Verification items for the finished model (mm, model axes). Face numbers are marked on the shaded views. A direction names the side the tool comes from. Round coordinates to 2 decimals unless told otherwise and drop trailing zeros. Loops run counter-clockwise (first coordinate to the right, second up) from the corner with the lowest first, then second, coordinate; pieces in that order, holes last.
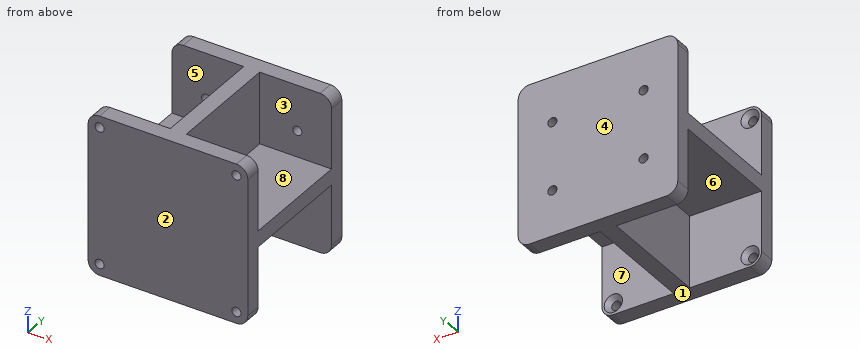
from build123d import *

# Parameters (mm, degrees)
SKETCH1_R           = 2
BOSS_EXTRUDE1_DEPTH = 3.5
BOSS_EXTRUDE2_DEPTH = 50
BOSS_EXTRUDE3_START = 7
SKETCH3_R           = 2
BOSS_EXTRUDE3_DEPTH = 7
CHAMFER1_SIZE       = 2


with BuildPart() as part:
    # Sketch1 → Boss-Extrude1 (new, symmetric)
    with BuildSketch(Plane(origin=(0, 0, 0), x_dir=(1, 0, 0), z_dir=(0, 1, 0))):
        with BuildLine():
            Line((-30, 35), (30, 35))
            ThreePointArc((30, 35), (33.535533906, 33.535533906), (35, 30))
            Line((35, 30), (35, -30))
            ThreePointArc((35, -30), (33.535533906, -33.535533906), (30, -35))
            Line((30, -35), (-30, -35))
            ThreePointArc((-30, -35), (-33.535533906, -33.535533906), (-35, -30))
            Line((-35, -30), (-35, 30))
            ThreePointArc((-35, 30), (-33.535533906, 33.535533906), (-30, 35))
        make_face()
        with Locations(Location((30, 30, 0), (0, 0, 270))):
            Circle(SKETCH1_R, mode=Mode.SUBTRACT)
        with Locations(Location((-30, 30, 0), (0, 0, 90))):
            Circle(SKETCH1_R, mode=Mode.SUBTRACT)
        with Locations(Location((30, -30, 0), (0, 0, 90))):
            Circle(SKETCH1_R, mode=Mode.SUBTRACT)
        with Locations(Location((-30, -30, 0), (0, 0, 270))):
            Circle(SKETCH1_R, mode=Mode.SUBTRACT)
    extrude(amount=BOSS_EXTRUDE1_DEPTH, both=True)

    # Sketch2 → Boss-Extrude2 (add)
    with BuildSketch(Plane(origin=(0, 3.5, 0), x_dir=(1, 0, 0), z_dir=(0, 1, 0))):
        Polygon((-3.5, 35), (3.5, 35), (3.5, 3.5), (35, 3.5), (35, -3.5), (3.5, -3.5), (3.5, -35), (-3.5, -35), (-3.5, -3.5), (-35, -3.5), (-35, 3.5), (-3.5, 3.5), align=None)
    extrude(amount=BOSS_EXTRUDE2_DEPTH)

    # Sketch3 → Boss-Extrude3 (add)
    with BuildSketch(Plane(origin=(0, 53.5, 0), x_dir=(1, 0, 0), z_dir=(0, 1, 0)).offset(BOSS_EXTRUDE3_START)):
        with BuildLine():
            Line((30, -35), (-30, -35))
            ThreePointArc((-30, -35), (-33.535533906, -33.535533906), (-35, -30))
            Line((-35, -30), (-35, 30))
            ThreePointArc((-35, 30), (-33.535533906, 33.535533906), (-30, 35))
            Line((-30, 35), (30, 35))
            ThreePointArc((30, 35), (33.535533906, 33.535533906), (35, 30))
            Line((35, 30), (35, -30))
            ThreePointArc((35, -30), (33.535533906, -33.535533906), (30, -35))
        make_face()
        with Locations(Location((20, -15, 0), (0, 0, 270))):
            Circle(SKETCH3_R, mode=Mode.SUBTRACT)
        with Locations(Location((20, 15, 0), (0, 0, 270))):
            Circle(SKETCH3_R, mode=Mode.SUBTRACT)
        with Locations(Location((-20, 15, 0), (0, 0, 90))):
            Circle(SKETCH3_R, mode=Mode.SUBTRACT)
        with Locations(Location((-20, -15, 0), (0, 0, 90))):
            Circle(SKETCH3_R, mode=Mode.SUBTRACT)
    extrude(amount=-BOSS_EXTRUDE3_DEPTH)

    # Chamfer1
    chamfer1_edges = [part.edges().sort_by_distance(p)[0] for p in [
        (30, 3.5, -32),
        (-30, 3.5, -28),
        (30, 3.5, 32),
        (-30, 3.5, 28),
    ]]
    chamfer(chamfer1_edges, length=CHAMFER1_SIZE)


solid = part.part
1. Release check for a two-part mould opening along Y. For the marked faces 1, 2, 3 and 4 record: released by +Y, released by -Y, zero draft, split by the parting line, or undercut.
2. Section check B-B (z = 15). Enter the section's corners in (x, y), then the cut area to 3 significant figures.
3. Scan lines: L1, parallel to Z at x = -20, y = 57.25; L2, parallel to X at y = -0.95, z = 30; L3, parallel to X at y = 58, z = 15. Record each from-to range of solid material in increasing order.
4. Section check C-C (x = -9.5). Enter the section's corners in (y, z), then the cut area to 3 significant figures.
5. Gauge pin test, flat ends, axial feed: P1, Ø4, axis at y = 21.5, z = -17, coming from the +X side; P2, Ø2.5, axis at x = 20, z = -15, coming from the +Y side; P3, Ø1.5, axis at y = 18.5, z = 25, coming from the -X side. Record the tip position at first contact, or that the pin passes through.
6. Section check D-D (y = 25). Enter the section's corners in (x, z).
7. Tool access check on the marked faces 5, 6, 7 and 8. Record the directions out of +Z, -Z, +X, -X, +Y, -Y that give a thin tool (end or side, any length) a straight path to the whole face; none if there is none.
8. Section check A-A (x = -20). Enter the section's corners in (y, z).
Taken from the geometry:
1. face 1: zero draft
1. face 2: released by -Y
1. face 3: undercut
1. face 4: released by +Y
2. outline: (-35, -3.5) - (35, -3.5) - (35, 3.5) - (3.5, 3.5) - (3.5, 53.5) - (18, 53.5) - (18, 60.5) - (-18, 60.5) - (-18, 53.5) - (-3.5, 53.5) - (-3.5, 3.5) - (-35, 3.5) - close; (-35, 53.5) - (-22, 53.5) - (-22, 60.5) - (-35, 60.5) - close; (22, 53.5) - (35, 53.5) - (35, 60.5) - (22, 60.5) - close
2. area: 1,270 mm2
3. L1: z = -35 to -17, -13 to 13, 17 to 35
3. L2: x = -35 to -32, -28 to 28, 32 to 35
3. L3: x = -35 to -22, -18 to 18, 22 to 35
4. outline: (-3.5, -35) - (3.5, -35) - (3.5, -3.5) - (53.5, -3.5) - (53.5, -35) - (60.5, -35) - (60.5, 35) - (53.5, 35) - (53.5, 3.5) - (3.5, 3.5) - (3.5, 35) - (-3.5, 35) - close
4. area: 1,330 mm2
5. P1: stops at x = 3.5
5. P2: stops at y = 3.5
5. P3: stops at x = -3.5
6. outline: (-35, -3.5) - (-3.5, -3.5) - (-3.5, -35) - (3.5, -35) - (3.5, -3.5) - (35, -3.5) - (35, 3.5) - (3.5, 3.5) - (3.5, 35) - (-3.5, 35) - (-3.5, 3.5) - (-35, 3.5) - close
7. face 5: +Z, -X
7. face 6: -Z, -X
7. face 7: -Z, +X
7. face 8: +Z, +X
8. outline: (-3.5, -35) - (3.5, -35) - (3.5, -3.5) - (53.5, -3.5) - (53.5, -13) - (60.5, -13) - (60.5, 13) - (53.5, 13) - (53.5, 3.5) - (3.5, 3.5) - (3.5, 35) - (-3.5, 35) - close; (53.5, -35) - (60.5, -35) - (60.5, -17) - (53.5, -17) - close; (53.5, 17) - (60.5, 17) - (60.5, 35) - (53.5, 35) - close
